Autodesk Inventor part; units mm, degrees
ref_plane "YZ Plane" through (0, 0, 0) normal (1, 0, 0) x (0, 1, 0)
ref_plane "XZ Plane" through (0, 0, 0) normal (0, 1, 0) x (-1, 0, 0)
ref_plane "XY Plane" through (0, 0, 0) normal (0, 0, 1) x (1, 0, 0)
sketch "Sketch1" plane through (0, 0, 0) normal (0, 1, 0) x (-1, 0, 0)
  line L0 (0, 0) -> (40, 0)
  line L1 (40, 0) -> (40, -40)
  line L2 (40, -40) -> (0, -40)
  line L3 (0, -40) -> (0, 0)
  dimension "d0" = 40
  dimension "d1" = 40
extrude "Extrusion1" add sketch "Sketch1" along normal blind 40
chamfer "Chamfer1" distance 4 angle 45 4 edges at (0, 20, 0) (0, 20, -40) (-40, 20, 0) (-40, 20, -40)
sketch "Sketch2" plane through (0, 40, 0) normal (0, 1, 0) x (1, 0, 0)
  circle A0 centre (-20, 20) radius 2.5
  line L0 (-40, 36) -> (-36, 40)
  line L1 (-40, 36) -> (-40, 4)
  line L2 (-36, 0) -> (-40, 4)
  line L3 (-36, 0) -> (-4, 0)
  line L4 (0, 4) -> (-4, 0)
  line L5 (0, 4) -> (0, 36)
  line L6 (-4, 40) -> (0, 36)
  line L7 (-4, 40) -> (-36, 40)
  point P0 (0, 0)
  dimension "d7" = 5
  dimension "d8" = 40
  dimension "d9" = 20
  dimension "d10" = 20
extrude "Extrusion2" add sketch "Sketch2" along normal blind 20 contours A0
sketch "Sketch3" plane through (0, 40, 0) normal (0, 1, 0) x (1, 0, 0)
  circle A0 centre (-20, 20) radius 2.5
  line L0 (-40, 36) -> (-36, 40)
  line L1 (-40, 36) -> (-40, 4)
  line L2 (-36, 0) -> (-40, 4)
  line L3 (-36, 0) -> (-4, 0)
  line L4 (0, 4) -> (-4, 0)
  line L5 (0, 4) -> (0, 36)
  line L6 (-4, 40) -> (0, 36)
  line L7 (-4, 40) -> (-36, 40)
  circle A1 centre (-4.5, 4.5) radius 1.75
  circle A2 centre (-4.5, 35.5) radius 1.75
  circle A3 centre (-35.5, 4.5) radius 1.75
  circle A4 centre (-35.5, 35.5) radius 1.75
  point P0 (0, 0)
  dimension "d13" = 3.5
  dimension "d15" = 4
  dimension "d17" = 40
  dimension "d20" = 31
  dimension "d23" = 31
  dimension "d28" = 4.5
  dimension "d29" = 4.5
extrude "Extrusion3" cut sketch "Sketch3" against normal blind 5 contours A1 | A2 | A3 | A4
equation "\"d10\" = d9"
equation "\"d28\" = -0.5 * d23 + 0.5 * d17"
equation "\"d29\" = d28"
properties part number "mOTOR" material "Acetal Resin, Black"
Could you check a few things on this model? Use its own coordinates, in mm. A direction names the side the tool comes from. Give positions to 0.01 mm unless a question says otherwise; leave off trailing zeros. Order: outer loops, then holes, each group sorted by start corner. A loop starts at its lowest first (then second) coordinate and runs counter-clockwise, first axis right, second up.
1. Suppose I cut it at D-D (y = 46.5). List the corners of the cut face in (x, z) for me, plus the area to 3 significant figures.
2. We'd pull the mould along Z, two halves only. Please class faces 3 (the flat face through (-2, 20, -2)), 4 (the cylindrical face through (-36.89, 37.53, -3.44)), 5 (the flat face through (-20, 20, -40)), 6 (the cylindrical face through (-4.88, 37.53, -33.79)): pulls with the +Z half, pulls with the -Z half, needs draft (parallel to the pull), parting line crosses it, or undercut.
3. Suppose I cut it at C-C (z = -20). List the corners of the cut face in (x, y) for me.
4. Suppose I cut it at A-A (y = 38). List the corners of the cut face in (x, z) for me.
5. Suppose I cut it at B-B (x = -20). List the corners of the cut face in (y, z) for me.
6. Will these pins go through, and if not, where does the flat tip stop? P1, Ø4.5, axis at x = -35.5, z = -4.5, coming from the +Y side; P2, Ø3, axis at x = -35.5, z = -35.5, coming from the -Y side; P3, Ø3, axis at x = -18, y = 50, coming from the +Z side; P4, Ø1, axis at x = -35, z = -35.5, coming from the +Y side.
7. I need wall thicknesses on L1, parallel to X at y = 38.3, z = -4.5; L2, parallel to X at y = 36.5, z = -37. Which ranges of each line are inside material? Lowest first, please.
8. For faces 1 (the flat face through (-20, 20, 0)), 2 (the flat face through (-5, 35, -5)), which set-ups out of +Z, -Z, +X, -X, +Y, -Y let a thin tool reach every point of the face, with its end or its side?
Solved:
1. outline: circle Ø5 at (-20, -20)
1. area: 19.6 mm2
2. face 3: pulls with the +Z half
2. face 4: undercut
2. face 5: pulls with the -Z half
2. face 6: undercut
3. outline: (-40, 0) - (0, 0) - (0, 40) - (-17.5, 40) - (-17.5, 60) - (-22.5, 60) - (-22.5, 40) - (-40, 40) - close
4. outline: (-40, -36) - (-36, -40) - (-4, -40) - (0, -36) - (0, -4) - (-4, 0) - (-36, 0) - (-40, -4) - close; hole circle Ø3.5 at (-35.5, -35.5); hole circle Ø3.5 at (-35.5, -4.5); hole circle Ø3.5 at (-4.5, -35.5); hole circle Ø3.5 at (-4.5, -4.5)
5. outline: (0, -40) - (40, -40) - (40, -22.5) - (60, -22.5) - (60, -17.5) - (40, -17.5) - (40, 0) - (0, 0) - close
6. P1: stops at y = 40
6. P2: stops at y = 0
6. P3: stops at z = -17.55
6. P4: stops at y = 35
7. L1: x = -40 to -37.25, -33.75 to -6.25, -2.75 to 0
7. L2: x = -39 to -36.4, -34.6 to -5.4, -3.6 to -1
8. face 1: +Z, +X, -X, +Y, -Y
8. face 2: +Y
